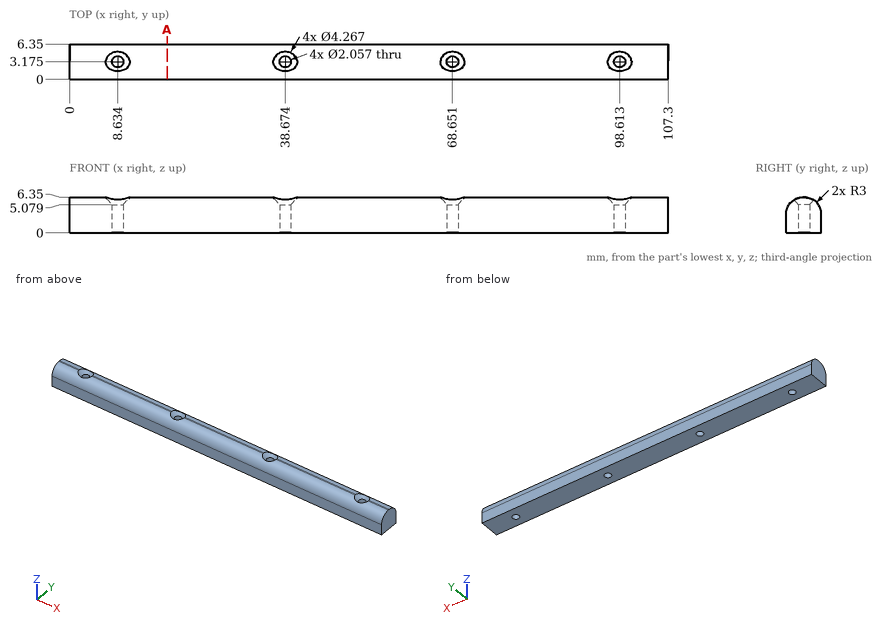
The drawing under review shows one solid part. Ordinate dimensions are in mm from its lowest x, y, z. Round coordinates to 2 decimals unless told otherwise and drop trailing zeros. Order: outer loops, then holes, each group sorted by start corner. A loop starts at its lowest first (then second) coordinate and runs counter-clockwise, first axis right, second up. Notation, with made-up numbers: M 83,28 L 88,28 A12 ccw 88,50 Z; hole C 73,-23.5 d5. An arc over 180 degrees is marked long. Answer as CSV lines item,"result". Start each with the question number.
1) Wall thickness on line 1 along X through (y, z) = (3.25, 3.5) (1 decimal); line 2 along X through (y, z) = (3.5, 5.5) (1 decimal); line 3 along Z through (x, y) = (87, 2.75): over which ranges is each line inside the solid? List them lowest first. Write a range as [from, to].
2) Add section A-A (x = 17.5). Give the boundary of the cut face in (y, z).
3) For pin 1 Ø1.6 at (x, y) = (68.65, 3.18) entering from +Z; pin 2 Ø2.5 at (x, y) = (38.67, 3.18) entering from +Z; pin 3 Ø3 at (x, z) = (16.5, 5) entering from -Y, all flat-tipped, find the tip position at first contact; note any pin that passes through.
Resolved:
1,line 1,"[0, 7.6], [9.7, 37.6], [39.7, 67.6], [69.7, 97.6], [99.6, 107.3]"
1,line 2,"[0, 7.3], [10, 37.3], [40, 67.3], [70, 97.3], [100, 107.3]"
1,line 3,"[0, 6.34]"
2,outline,"M 0,0 L 6.35,0 L 6.35,3.35 A3 ccw 3.35,6.35 L 3,6.35 A3 ccw 0,3.35 Z"
3,pin 1,"through"
3,pin 2,"z = 5.34"
3,pin 3,"y = 0"
